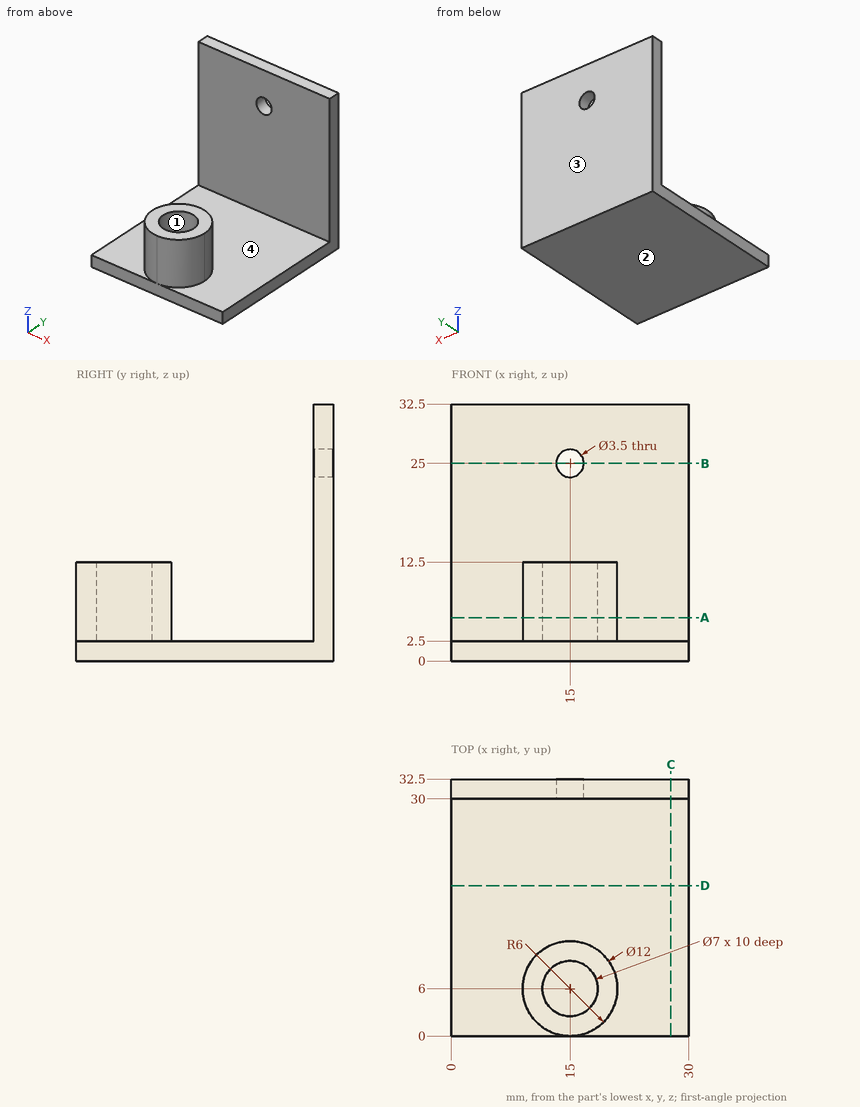
Drawing for the job (mm, zero at the part's lowest x, y, z). Give positions to 0.01 mm unless a question says otherwise; leave off trailing zeros. Order: outer loops, then holes, each group sorted by start corner. A loop starts at its lowest first (then second) coordinate and runs counter-clockwise, first axis right, second up. Notation, with made-up numbers: (-16, 28) -> (37, 28) arc R19 ccw to (37, 57) -> close; hole circle Ø3 at (-9, 53.25). An arc over 180 degrees is marked (long way). Use one line per item in the form item = value.
(1) Saw through at C-C (x = 27.75). Write the cut outline in (y, z), then the cut area to 3 significant figures.
Solution:
outline = (0, 0) -> (32.5, 0) -> (32.5, 32.5) -> (30, 32.5) -> (30, 2.5) -> (0, 2.5) -> close
area = 156 mm²
(2) Flat gauge pins, fed straight in: P1, Ø2, axis at x = 15, z = 25, coming from the -Y side; P2, Ø15, axis at x = 10.5, y = 14, coming from the +Z side; P3, Ø12, axis at x = 27, y = 12.5, coming from the +Z side; P4, Ø8, axis at y = 8.5, z = 13.5, coming from the -X side. Where does each tip first touch, or does it go through?
Solution:
P1 = through
P2 = 12.5
P3 = 2.5
P4 = 9
(3) Saw through at A-A (z = 5.5). Write the cut outline in (x, y).
Solution:
outline = (0, 30) -> (30, 30) -> (30, 32.5) -> (0, 32.5) -> close; circle Ø12 at (15, 6); hole circle Ø7 at (15, 6)
(4) Drill centre lines: line 1 (Z direction, x = 15, y = 31.65); line 2 (X direction, y = 6, z = 9.5); line 3 (Z direction, x = 25.25, y = 3.5). Where is each one in solid material? Low to high. Write a range as from..to.
Solution:
line_1 = 0..23.25, 26.75..32.5
line_2 = 9..11.5, 18.5..21
line_3 = 0..2.5
(5) Saw through at D-D (y = 19). Write the cut outline in (x, z).
Solution:
outline = (0, 0) -> (30, 0) -> (30, 2.5) -> (0, 2.5) -> close
(6) Saw through at B-B (z = 25). Write the cut outline in (x, y).
Solution:
outline = (0, 30) -> (13.25, 30) -> (13.25, 32.5) -> (0, 32.5) -> close; (16.75, 30) -> (30, 30) -> (30, 32.5) -> (16.75, 32.5) -> close
(7) Pull direction Y, two halves, no side cores. Call the marked faces 1, 2, 3 and 4: +Y half, -Y half, draft (parallel to the pull), parting line (faces both ways), or undercut.
Solution:
face_1 = undercut
face_2 = draft
face_3 = +Y half
face_4 = undercut
